Geometry: final body of the model. Coordinates: model frame, mm. A direction names the side the tool comes from. Give positions to 0.01 mm unless a question says otherwise; leave off trailing zeros. Order: outer loops, then holes, each group sorted by start corner. A loop starts at its lowest first (then second) coordinate and runs counter-clockwise, first axis right, second up. Notation, with made-up numbers: (9, 67.25) - (23, 67.25) arc R17 cw to (23, 88.25) - close; hole circle Ø11 at (41.5, 63). An arc over 180 degrees is marked (long way). Use one line per item in the form item = value.
from build123d import *

# Parameters (mm, degrees)
SKETCH3_W           = 38
SKETCH3_H           = 34
SKETCH3_W_2         = 26
SKETCH3_H_2         = 22
BOSS_EXTRUDE1_DEPTH = 22
SKETCH4_W           = 24
SKETCH4_H           = 22
BOSS_EXTRUDE2_DEPTH = 1
SKETCH5_R           = 2.65
CUT_EXTRUDE1_DEPTH  = 12
SKETCH7_R           = 5.65
CUT_EXTRUDE3_DEPTH  = 4.2
SKETCH8_R           = 6.15
CUT_EXTRUDE4_DEPTH  = 57.151580565
SKETCH9_R           = 9.15
CUT_EXTRUDE5_DEPTH  = 4.2
SKETCH10_R          = 9.15
CUT_EXTRUDE6_DEPTH  = 4.2
SKETCH15_R          = 1.8
CUT_EXTRUDE7_DEPTH  = 57.151580565
FILLET1_R           = 3
FILLET3_R           = 2.5
FILLET4_R           = 2.2
FILLET5_R           = 2.4


with BuildPart() as part:
    # Sketch3 → Boss-Extrude1 (new body)
    with BuildSketch(Plane(origin=(0, 0, 0), x_dir=(1, 0, 0), z_dir=(0, 1, 0))):
        with Locations((19, -17)):
            Rectangle(SKETCH3_W, SKETCH3_H)
        with Locations((19, -17)):
            Rectangle(SKETCH3_W_2, SKETCH3_H_2, mode=Mode.SUBTRACT)
    extrude(amount=BOSS_EXTRUDE1_DEPTH)

    # Sketch4 → Boss-Extrude2 (add)
    with BuildSketch(Plane.XY.offset(34)):
        with Locations((19, 11)):
            Rectangle(SKETCH4_W, SKETCH4_H)
    extrude(amount=BOSS_EXTRUDE2_DEPTH)

    # Sketch5 → Cut-Extrude1 (cut)
    with BuildSketch(Plane.XY.offset(35)):
        with Locations((19, 11)):
            Circle(SKETCH5_R)
    extrude(amount=-CUT_EXTRUDE1_DEPTH, mode=Mode.SUBTRACT)

    # Sketch7 → Cut-Extrude3 (cut)
    with BuildSketch(Plane(origin=(0, 0, 28), x_dir=(-1, 0, 0), z_dir=(0, 0, -1))):
        with Locations((-19, 11)):
            Circle(SKETCH7_R)
    extrude(amount=-CUT_EXTRUDE3_DEPTH, mode=Mode.SUBTRACT)

    # Sketch8 → Cut-Extrude4 (cut, through all)
    with BuildSketch(Plane(origin=(38, 0, 0), x_dir=(0, 0, -1), z_dir=(1, 0, 0))):
        with Locations((-15, 11)):
            Circle(SKETCH8_R)
    extrude(amount=-CUT_EXTRUDE4_DEPTH, mode=Mode.SUBTRACT)

    # Sketch9 → Cut-Extrude5 (cut)
    with BuildSketch(Plane(origin=(6, 0, 0), x_dir=(0, 0, -1), z_dir=(1, 0, 0))):
        with Locations((-15, 11)):
            Circle(SKETCH9_R)
    extrude(amount=-CUT_EXTRUDE5_DEPTH, mode=Mode.SUBTRACT)

    # Sketch10 → Cut-Extrude6 (cut)
    with BuildSketch(Plane(origin=(38, 0, 0), x_dir=(0, 0, -1), z_dir=(1, 0, 0))):
        with Locations((-15, 11)):
            Circle(SKETCH10_R)
    extrude(amount=-CUT_EXTRUDE6_DEPTH, mode=Mode.SUBTRACT)

    # Sketch15 → Cut-Extrude7 (cut, through all)
    with BuildSketch(Plane(origin=(0, 0, 0), x_dir=(-1, 0, 0), z_dir=(0, -1, 0))):
        with Locations(Location((-4, -30, 0), (0, 0, 90))):
            Circle(SKETCH15_R)
        with Locations(Location((-34, -30, 0), (0, 0, 90))):
            Circle(SKETCH15_R)
        with Locations(Location((-34, -4, 0), (0, 0, 90))):
            Circle(SKETCH15_R)
        with Locations(Location((-4, -4, 0), (0, 0, 90))):
            Circle(SKETCH15_R)
    extrude(amount=-CUT_EXTRUDE7_DEPTH, mode=Mode.SUBTRACT)

    # Fillet1
    # the kernel refuses this fillet: 3 mm, written as the material it takes off along each edge
    with BuildSketch(Plane(origin=(38, -7.5, 0), x_dir=(-1, 0, 0), z_dir=(0, 1, 0)), Plane(origin=(38, -7.5, 34), x_dir=(0, 0, -1), z_dir=(0, 1, 0))) as fillet1_piece_1:
        with BuildLine():
            CenterArc((FILLET1_R, FILLET1_R), FILLET1_R, 180, 90)
            Line((0, FILLET1_R), (-FILLET1_R * 0.02, FILLET1_R))
            Line((-FILLET1_R * 0.02, FILLET1_R), (-FILLET1_R * 0.02, -FILLET1_R * 0.02))
            Line((-FILLET1_R * 0.02, -FILLET1_R * 0.02), (FILLET1_R, -FILLET1_R * 0.02))
            Line((FILLET1_R, -FILLET1_R * 0.02), (FILLET1_R, 0))
        make_face()
    extrude(amount=37, mode=Mode.SUBTRACT)
    with BuildSketch(Plane(origin=(7, -5.590169944, 35), x_dir=(0, 0, -1), z_dir=(0, 1, 0)), Plane(origin=(31, 27.590169944, 35), x_dir=(0, 0, -1), z_dir=(0, -1, 0))) as fillet1_piece_2:
        with BuildLine():
            CenterArc((3, -2.236067977), FILLET1_R, 131.810314896, 48.189685104)
            Line((0, -2.236067977), (-0.06, -2.236067977))
            Line((-0.06, -2.236067977), (-0.06, 0))
            Line((-0.06, 0), (0, 0.06))
            ThreePointArc((0, 0.06), (0.5, 0.06), (0.96, 0.04472136))
            Line((0.96, 0.04472136), (1, 0))
        make_face()
    extrude(amount=33.180339887, mode=Mode.SUBTRACT)
    with BuildSketch(Plane(origin=(0, -7.5, 34), x_dir=(0, 0, -1), z_dir=(0, 1, 0)), Plane(origin=(0, -7.5, 0), x_dir=(1, 0, 0), z_dir=(0, 1, 0))) as fillet1_piece_3:
        with BuildLine():
            CenterArc((FILLET1_R, -FILLET1_R), FILLET1_R, 90, 90)
            Line((0, -FILLET1_R), (-FILLET1_R * 0.02, -FILLET1_R))
            Line((-FILLET1_R * 0.02, -FILLET1_R), (-FILLET1_R * 0.02, FILLET1_R * 0.02))
            Line((-FILLET1_R * 0.02, FILLET1_R * 0.02), (FILLET1_R, FILLET1_R * 0.02))
            Line((FILLET1_R, FILLET1_R * 0.02), (FILLET1_R, 0))
        make_face()
    extrude(amount=37, mode=Mode.SUBTRACT)

    # Fillet3
    fillet3_edges = [part.edges().sort_by_distance(p)[0] for p in [
        (6, 11, 28),
        (32, 11, 6),
    ]]
    fillet(fillet3_edges, radius=FILLET3_R)

    # Fillet4
    fillet4_edges = [part.edges().sort_by_distance(p)[0] for p in [
        (32, 11, 28),
    ]]
    fillet(fillet4_edges, radius=FILLET4_R)

    # Fillet5
    # the kernel refuses this fillet: 2.4 mm, written as the material it adds along each edge
    with BuildSketch(Plane(origin=(6, 6.65, 6), x_dir=(0, 0, 1), z_dir=(0, 1, 0))) as fillet5_piece_1_section:
        with BuildLine():
            CenterArc((FILLET5_R, FILLET5_R), FILLET5_R, 180, 90)
            Line((0, FILLET5_R), (0, 0))
            Line((0, 0), (FILLET5_R, 0))
        make_face()
    fillet5_piece_1 = extrude(amount=15.35, mode=Mode.PRIVATE)
    fillet5_piece_1 = fillet5_piece_1 - Plane(origin=(6.746267067, 11, 15), x_dir=(0, 0, -1), z_dir=(1, 0, 0)) * Cylinder(9.15, 41, mode=Mode.PRIVATE)
    add(fillet5_piece_1)
    with BuildSketch(Plane(origin=(6, 0, 6), x_dir=(0, 0, 1), z_dir=(0, 1, 0))) as fillet5_piece_2_section:
        with BuildLine():
            CenterArc((FILLET5_R, FILLET5_R), FILLET5_R, 180, 90)
            Line((0, FILLET5_R), (0, 0))
            Line((0, 0), (FILLET5_R, 0))
        make_face()
    fillet5_piece_2 = extrude(amount=15.35, mode=Mode.PRIVATE)
    fillet5_piece_2 = fillet5_piece_2 - Plane(origin=(6.573929996, 11, 15), x_dir=(0, 0, -1), z_dir=(1, 0, 0)) * Cylinder(9.15, 41, mode=Mode.PRIVATE)
    add(fillet5_piece_2)


solid = part.part
(1) Cut plane B-B on z = 4. Output: boundary loops of the cut face in (x, y), plus the area to 3 significant figures.
Computed values:
outline = (0, 0) - (2.2, 0) - (2.2, 22) - (0, 22) - close; (5.8, 0) - (32.2, 0) - (32.2, 22) - (5.8, 22) - close; (35.8, 0) - (38, 0) - (38, 22) - (35.8, 22) - close
area = 678 mm²
(2) Cut plane D-D on z = 30. Output: boundary loops of the cut face in (x, y).
Computed values:
outline = (0, 0) - (2.2, 0) - (2.2, 22) - (0, 22) - close; (5.8, 0) - (32.2, 0) - (32.2, 22) - (5.8, 22) - close; (35.8, 0) - (38, 0) - (38, 22) - (35.8, 22) - close; hole circle Ø11.3 at (19, 11)
(3) Reachability of faces 1 (the face through (32, 8, 21)), 2 (the face through (33, 11, 34)), 3 (the face through (21.45, 9.99, 33.62)), 4 (the face through (4.413, 13.748, 6.273)) from +Z, -Z, +X, -X, +Y, -Y: full face, straight path, thin tool, end or side. Return the list, or none.
Computed values:
face_1 = +Y, -Y
face_2 = +Z, +X, +Y, -Y
face_3 = +Z
face_4 = none
(4) Cut plane C-C on x = 12.5. Output: boundary loops of the cut face in (y, z).
Computed values:
outline = (0, 0) - (22, 0) - (22, 6) - (0, 6) - close; (0, 28) - (22, 28) - (22, 35) - (0, 35) - close
(5) Cut plane A-A on x = 4. Output: boundary loops of the cut face in (y, z), plus the area to 3 significant figures.
Computed values:
outline = (0, 0) - (22, 0) - (22, 2.2) - (0, 2.2) - close; (0, 5.8) - (22, 5.8) - (22, 28.2) - (0, 28.2) - close; (0, 31.8) - (22, 31.8) - (22, 34) - (0, 34) - close; hole circle Ø18.3 at (11, 15)
area = 327 mm²
(6) Pull-direction query (Z, two-part tool) for faces 5 (the face through (37.14, 10.85, 0.9)), 6 (the face through (19, 0, 29)), 7 (the face through (34.541, 10.846, 28.283)); classes: released by +Z, released by -Z, zero draft, split by the parting line, or undercut.
Computed values:
face_5 = released by -Z
face_6 = zero draft
face_7 = undercut
(7) Ray query, line 1 along X through (y, z) = (17.25, 16); line 2 along Z through (x, y) = (4.5, 20.75); line 3 along Z through (x, y) = (10.5, 9). Return the intervals inside material, ascending.
Computed values:
line_1 = 0 to 1.8, 32 to 33.8
line_2 = 0 to 2.27, 5.73 to 28.27, 31.73 to 34
line_3 = 0 to 6, 28 to 35
(8) Contact query for a flat-ended pin moving along its axis: pin 1 Ø1.2 at (x, y) = (33, 11.5) entering from +Z. Output: stop coordinate, or through.
Computed values:
pin_1 = 34
